from build123d import *

# Parameters (mm, degrees)
F0_W = 3.175
F0_H = 1.5875


with BuildPart() as f2:
    # F2: sweep along a path in F1
    with BuildLine(Plane.YZ) as f2_path:
        Line((0, 0), (0, 50.8))
        ThreePointArc((0, 50.8), (0.4280140937, 54.0549830382), (1.6829564702, 57.0886656642))
        ThreePointArc((1.6829564702, 57.0886656642), (4.7221119441, 57.1776447605), (7.5789801776, 56.1371222138))
        ThreePointArc((7.5789801776, 56.1371222138), (8.8392841167, 53.5932413011), (8.331840375, 50.8))
        ThreePointArc((8.331840375, 50.8), (6.5820659855, 50.2648305913), (4.7563990811, 50.3875378201))
    # F0 (on Top) → F2 (sweep)
    with BuildSketch(Plane.XY):
        Rectangle(F0_W, F0_H)
    sweep(path=f2_path.line, transition=Transition.RIGHT)


solid = f2.part
Geometry: final body of the model. Coordinates: model frame, mm. Coordinates: 2 decimals unless noted, no trailing zeros. Loops run counter-clockwise (first coordinate to the right, second up) from the corner with the lowest first, then second, coordinate; pieces in that order, holes last. Notation, with made-up numbers: (64.25, -32.75) - (116.25, -32.75) arc R25 ccw to (116.25, -6.75) - close; hole circle Ø9 at (-31.75, 46). An arc over 180 degrees is marked (long way). Put each result on its own line as item: value. Start each with the question number.
Q1. Cut plane A-A, the plane z = 37.5. Return loops of the section in (x, y), and give its area (3 significant figures).
Q2. Line query: line 1 (Y direction, x = 1.05, z = 47.5); line 2 (Y direction, x = -1, z = 50.5) (3 decimals); line 3 (Z direction, x = 0.45, y = 5). Output: solid intervals per line, ascending.
Q3. Pin query (flat end, axial travel): pin 1 Ø4 at (y, z) = (3.5, 47.5) entering from +X; pin 2 Ø1 at (x, z) = (0, 35.5) entering from +Y; pin 3 Ø1.5 at (x, y) = (-0.5, 8) entering from +Z. Return the tip coordinate at first contact, or that it passes through.
Q4. Pull-direction query (Z, two-part tool) for faces 1 (the flat face through (0.02, 4.76, 50.4)), 2 (the flat face through (0, 0.794, 26)), 3 (the flat face through (0, 0, 0)); classes: released by +Z, released by -Z, zero draft, split by the parting line, or undercut.
Filled sheet:
1. outline: (-1.59, -0.79) - (1.59, -0.79) - (1.59, 0.79) - (-1.59, 0.79) - close
1. area: 5.04 mm²
2. line 1: -0.79 to 0.79
2. line 2: -0.794 to 0.794, 4.785 to 9.071
2. line 3: 49.52 to 51.14, 56.32 to 57.94
3. pin 1: through
3. pin 2: y = 0.79
3. pin 3: z = 57.21
4. face 1: undercut
4. face 2: zero draft
4. face 3: released by -Z
